Could you check a few things on this drawing? It's one solid part, dimensions in mm from its lowest x, y, z. Coordinates: 2 decimals unless noted, no trailing zeros. Write each loop counter-clockwise with the first axis right and the second up, starting at its lowest first coordinate (ties: lowest second). Pieces come first, ordered by that corner, then holes. Notation, with made-up numbers: (-18, 80.25) - (10, 80.25) arc R15 ccw to (10, 84.25) - close; hole circle Ø8 at (14.5, -14). An arc over 180 degrees is marked (long way). Answer as a JSON object with one key per item and string values. Group by question number.
1) Will this pin go through, and if not, where does the flat tip stop? pin 1 Ø2.5 at (x, z) = (13.5, 22.5) entering from +Y.
2) If we section it at A-A (x = 13.5): Write out the boundary of the cut face in (y, z), plus the area to 3 significant figures.
3) If we section it at B-B (y = 1.7): State how many separate pieces and enclosed holes the cut face has, plus the area to 3 significant figures.
4) If we section it at D-D (z = 14.25): Write out the boundary of the cut face in (x, y), plus the area to 3 significant figures.
5) We'd pull the mould along X, two halves only. Please class the marked faces 1, 2 and 3: released by +X, released by -X, zero draft, split by the parting line, or undercut.
6) Please list where these lines run through material, in increasing order: line 1 along X through (y, z) = (0.75, 13.5); line 2 along Z through (x, y) = (7, 1.1); line 3 along X through (y, z) = (0.8, 20.5).
7) If we section it at C-C (x = 3.5): Write out the boundary of the cut face in (y, z), plus the area to 3 significant figures.
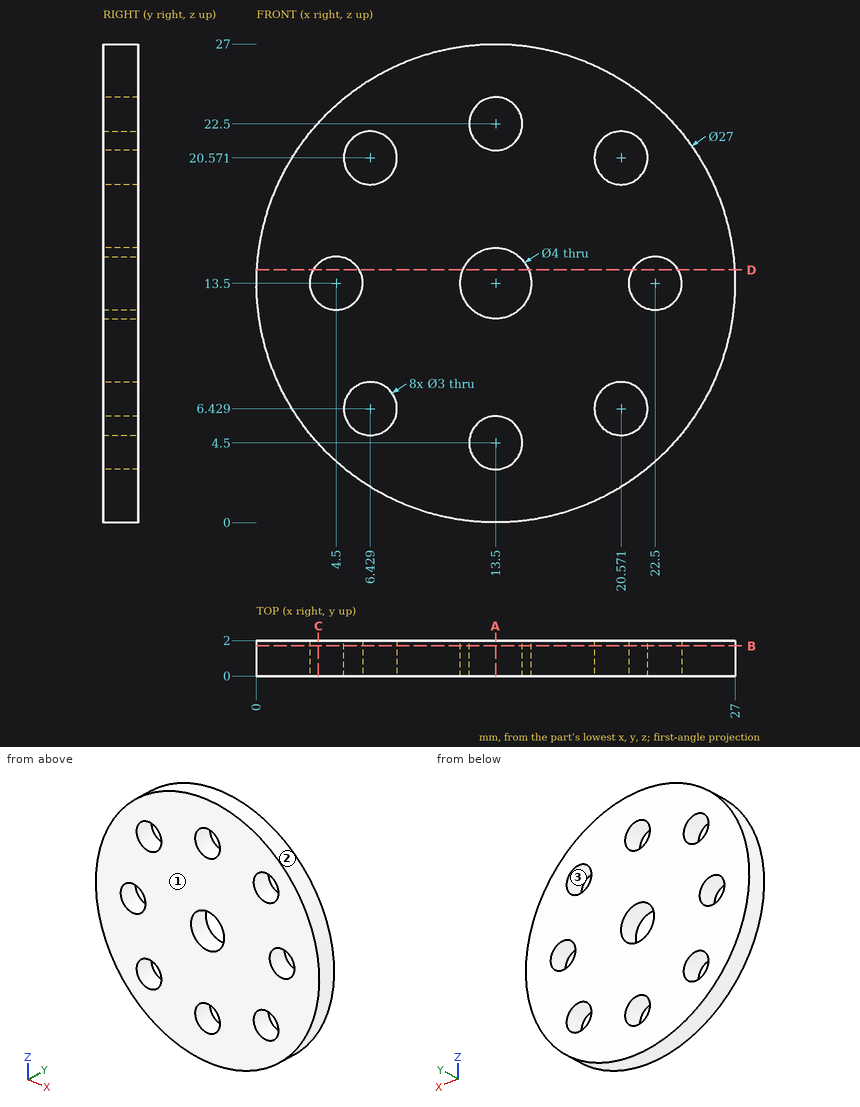
Here are the results:
{
 "1": {"pin 1": "passes through"},
 "2": {"outline": "(0, 0) - (2, 0) - (2, 3) - (0, 3) - close; (0, 6) - (2, 6) - (2, 11.5) - (0, 11.5) - close; (0, 15.5) - (2, 15.5) - (2, 21) - (0, 21) - close; (0, 24) - (2, 24) - (2, 27) - (0, 27) - close", "area": "34.0 mm²"},
 "3": {"separate pieces": "1", "enclosed holes": "9", "area": "503 mm²"},
 "4": {"outline": "(0.02, 0) - (3.2, 0) - (3.2, 2) - (0.02, 2) - close; (5.8, 0) - (11.65, 0) - (11.65, 2) - (5.8, 2) - close; (15.35, 0) - (21.2, 0) - (21.2, 2) - (15.35, 2) - close; (23.8, 0) - (26.98, 0) - (26.98, 2) - (23.8, 2) - close", "area": "36.1 mm²"},
 "5": {"face 1": "zero draft", "face 2": "split by the parting line", "face 3": "undercut"},
 "6": {"line 1": "x = 0 to 3, 6 to 11.5, 15.5 to 21, 24 to 27", "line 2": "z = 1.67 to 5.04, 7.82 to 19.18, 21.96 to 25.33", "line 3": "x = 1.96 to 4.93, 7.93 to 19.07, 22.07 to 25.04"},
 "7": {"outline": "(0, 4.43) - (2, 4.43) - (2, 12.38) - (0, 12.38) - close; (0, 14.62) - (2, 14.62) - (2, 22.57) - (0, 22.57) - close", "area": "31.8 mm²"}
}
